Input: dimensioned drawing with shaded views. Units: mm. Origin: part minimum x, y, z. A direction names the side the tool comes from. Round coordinates to 2 decimals unless told otherwise and drop trailing zeros. Loops run counter-clockwise (first coordinate to the right, second up) from the corner with the lowest first, then second, coordinate; pieces in that order, holes last. Notation, with made-up numbers: M -1,86.5 L 49,86.5 A36 cw 49,124.5 Z; hole C -25.75,88 d10. An arc over 180 degrees is marked long. Answer as a JSON object with one key per item and string values.
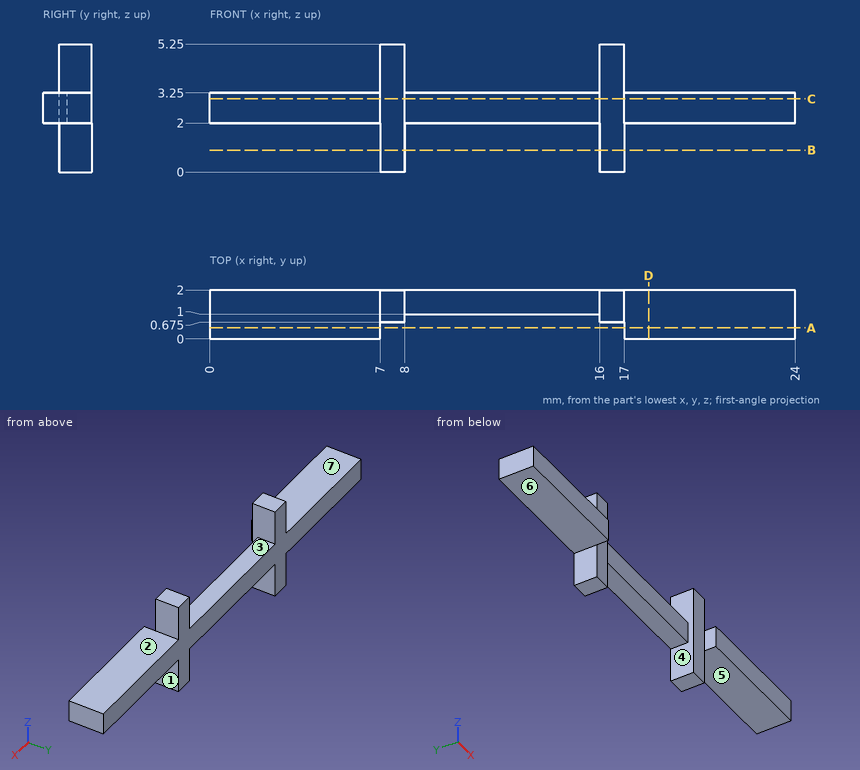
Item 1: Pull-direction query (X, two-part tool) for the marked faces 1, 2, 3 and 4; classes: pulls with the +X half, pulls with the -X half, needs draft (parallel to the pull), parting line crosses it, or undercut.
Answer sheet:
{"face 1": "pulls with the +X half", "face 2": "needs draft", "face 3": "undercut", "face 4": "undercut"}
Item 2: Line query: probe 1 along X at (y, z) = (1.35, 4.55); probe 2 along Z at (x, y) = (2, 0.55); probe 3 along Y at (x, z) = (14, 2.45). Output: solid intervals per line, ascending. Write a range as from..to.
Answer sheet:
{"probe 1": "x = 7..8, 16..17", "probe 2": "z = 2..3.25", "probe 3": "y = 1..2"}
Item 3: Section B-B on z = 0.9. Return the cut outline in (x, y) (3 decimals), then the cut area to 3 significant figures.
Answer sheet:
{"outline": "M 7,0.675 L 8,0.675 L 8,2 L 7,2 Z; M 16,0.675 L 17,0.675 L 17,2 L 16,2 Z", "area": "2.65 mm²"}
Item 4: Section D-D on x = 18. Return the cut outline in (y, z).
Answer sheet:
{"outline": "M 0,2 L 2,2 L 2,3.25 L 0,3.25 Z"}
Item 5: Contact query for flat-ended pins moving along their axis: pin 1 Ø0.7 at (y, z) = (1, 4) entering from -X; pin 2 Ø0.6 at (x, z) = (14, 2.5) entering from -Y; pin 3 Ø1.1 at (y, z) = (1.5, 4) entering from +X. Output: stop coordinate, or through.
Answer sheet:
{"pin 1": "stops at x = 7", "pin 2": "stops at y = 1", "pin 3": "stops at x = 17"}
Item 6: Section A-A on y = 0.45. Return the cut outline in (x, z), then the cut area to 3 significant figures.
Answer sheet:
{"outline": "M 0,2 L 7,2 L 7,3.25 L 0,3.25 Z; M 17,2 L 24,2 L 24,3.25 L 17,3.25 Z", "area": "17.5 mm²"}
Item 7: Section C-C on z = 3. Return the cut outline in (x, y) (3 decimals).
Answer sheet:
{"outline": "M 0,0 L 7,0 L 7,0.675 L 8,0.675 L 8,1 L 16,1 L 16,0.675 L 17,0.675 L 17,0 L 24,0 L 24,2 L 0,2 Z"}
Item 8: Access query for the marked faces 5, 6 and 7. Directions: +Z, -Z, +X, -X, +Y, -Y. A direction counts if a zero-diameter tool reaches every point of the face in a straight line with its end or side. Return the directions, or none.
Answer sheet:
{"face 5": "-Z, +X, +Y, -Y", "face 6": "-Z, -X, +Y, -Y", "face 7": "+Z, -X, +Y, -Y"}
